The listing builds one solid part. Answer for the finished solid, in the listing's coordinates (mm). Face numbers are marked on the shaded views. Coordinates: 2 decimals unless noted, no trailing zeros. Write each loop counter-clockwise with the first axis right and the second up, starting at its lowest first coordinate (ties: lowest second). Pieces come first, ordered by that corner, then holes.
from build123d import *

# Parameters (mm, degrees)
SKETCH1_R           = 6.35
BOSS_EXTRUDE1_DEPTH = 5.08
BOSS_EXTRUDE2_START = 38.1
SKETCH2_R           = 6.35
BOSS_EXTRUDE2_DEPTH = 38.1
FILLET1_R           = 0.508


with BuildPart() as part:
    # Sketch1 → Boss-Extrude1 (new body)
    with BuildSketch(Plane(origin=(0, 0, 0), x_dir=(1, 0, 0), z_dir=(0, 1, 0))):
        with Locations(Location((0, 0, 0), (0, 0, 270))):
            Circle(SKETCH1_R)
        with BuildLine():
            ThreePointArc((-1.27, 4.0132), (-5.2832, 0), (-1.27, -4.0132))
            Line((-1.27, -4.0132), (1.27, -4.0132))
            ThreePointArc((1.27, -4.0132), (5.2832, 0), (1.27, 4.0132))
            Line((1.27, 4.0132), (-1.27, 4.0132))
        make_face(mode=Mode.SUBTRACT)
    extrude(amount=BOSS_EXTRUDE1_DEPTH)

    # Sketch2 → Boss-Extrude2 (add)
    with BuildSketch(Plane.XZ.offset(BOSS_EXTRUDE2_START)):
        with Locations(Location((0, 0, 0), (0, 0, 270))):
            Circle(SKETCH2_R)
    extrude(amount=-BOSS_EXTRUDE2_DEPTH)

    # Fillet1
    fillet1_edges = [part.edges().sort_by_distance(p)[0] for p in [
        (0, 5.08, -4.0132),
        (5.2832, 5.08, 0),
        (0, -38.1, 6.35),
        (0, 5.08, 4.0132),
        (0, 5.08, -6.35),
        (-5.2832, 5.08, 0),
        (0, 0, 4.0132),
        (5.2832, 0, 0),
        (0, 0, -4.0132),
        (-5.2832, 0, 0),
    ]]
    fillet(fillet1_edges, radius=FILLET1_R)


solid = part.part
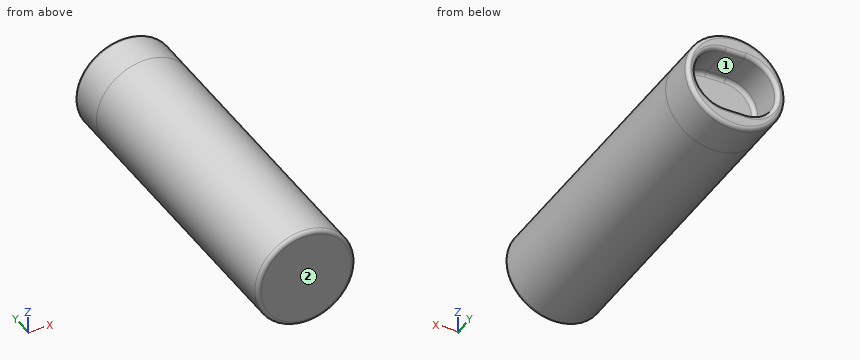
Q1. Find the intervals of material crossed by probe 1 along Y at (x, z) = (2, -3); probe 2 along Z at (x, y) = (-2.5, -28), in increasing order.
Answers below:
probe 1: y = -38.1 to 0
probe 2: z = -5.84 to 5.84
Q2. The part is cut by section A-A, the plane x = 0. Write down the section's boundary in (y, z).
Answers below:
outline: (-38.1, -5.84) arc R0.51 ccw to (-37.59, -6.35) - (4.57, -6.35) arc R0.51 ccw to (5.08, -5.84) - (5.08, -4.52) arc R0.51 ccw to (4.57, -4.01) - (0.51, -4.01) arc R0.51 cw to (0, -3.51) - (0, 3.51) arc R0.51 cw to (0.51, 4.01) - (4.57, 4.01) arc R0.51 ccw to (5.08, 4.52) - (5.08, 5.84) arc R0.51 ccw to (4.57, 6.35) - (-37.59, 6.35) arc R0.51 ccw to (-38.1, 5.84) - close
Q3. The part is cut by section C-C, the plane y = 2. Write down the section's boundary in (x, z).
Answers below:
outline: circle Ø12.7 at (0, 0); hole (-1.27, -4.01) - (1.27, -4.01) arc R4.01 ccw to (1.27, 4.01) - (-1.27, 4.01) arc R4.01 ccw to start
Q4. Given pin 1 (3 mm diameter, centred on x = 3, y = -10.5, fed in from -Z); pin 2 (2 mm diameter, centred on x = 0.5, y = 2, fed in from -Z); pin 3 (1.5 mm diameter, centred on y = -4.5, z = -2, fed in from +X); pin 4 (6 mm diameter, centred on x = -5, y = -14.5, fed in from +Z), each flat-ended and moving along its own axis, determine where each tip first touches the part or whether it passes through.
Answers below:
pin 1: stops at z = -6.17
pin 2: stops at z = -6.35
pin 3: stops at x = 6.23
pin 4: stops at z = 6.03
Q5. Determine the mould class of the marked faces 1 and 2 for opening direction Z: released by +Z, released by -Z, zero draft, split by the parting line, or undercut.
Answers below:
face 1: undercut
face 2: zero draft
Q6. The part is cut by section B-B, the plane z = 0. Write down the section's boundary in (x, y).
Answers below:
outline: (-6.35, -37.59) arc R0.51 ccw to (-5.84, -38.1) - (5.84, -38.1) arc R0.51 ccw to (6.35, -37.59) - (6.35, 4.57) arc R0.51 ccw to (5.84, 5.08) - (5.79, 5.08) arc R0.51 ccw to (5.28, 4.57) - (5.28, 0.51) arc R0.51 cw to (4.78, 0) - (-4.78, 0) arc R0.51 cw to (-5.28, 0.51) - (-5.28, 4.57) arc R0.51 ccw to (-5.79, 5.08) - (-5.84, 5.08) arc R0.51 ccw to (-6.35, 4.57) - close
